Input: part model. Units: mm. Frame: model coordinates. Face numbers are marked on the shaded views. Round coordinates to 2 decimals unless told otherwise and drop trailing zeros. Loops run counter-clockwise (first coordinate to the right, second up) from the corner with the lowest first, then second, coordinate; pieces in that order, holes last. Notation, with made-up numbers: (57, -20) -> (75, -20) arc R28 cw to (75, 19) -> close; hole circle Ø1 at (39, 67.5). An arc over 180 degrees is marked (long way). Answer in a Markdown table with one row per item. Add a question column.
Q1. Section C-C, the plane x = 5.5. Output: boundary loops of the cut face in (y, z).
Q2. Pin query (flat end, axial travel): pin 1 (2.5 mm diameter, centred on x = 0.5, y = 1, fed in from +Z); pin 2 (6 mm diameter, centred on x = -10, y = -6.5, fed in from +Z); pin 3 (12 mm diameter, centred on x = -8.5, z = 38, fed in from -Y). Return the tip coordinate at first contact, or that it passes through.
Q3. Mould query, pull axis Z, two halves, no side actions, for the marked faces 1 and 2. Classes: pulls with the +Z half, pulls with the -Z half, needs draft (parallel to the pull), parting line crosses it, or undercut.
Q4. Section A-A, the plane y = 0. Output: boundary loops of the cut face in (x, z).
Q5. Ray query, L1, parallel to Z at x = -4, y = 12.5; L2, parallel to Z at x = 11.5, y = -2.5; L3, parallel to Z at x = -5.5, y = -5.5. Return the intervals inside material, ascending. Write a range as from..to.
Q6. Section D-D, the plane y = 4. Output: boundary loops of the cut face in (x, z), and give its area (3 significant figures).
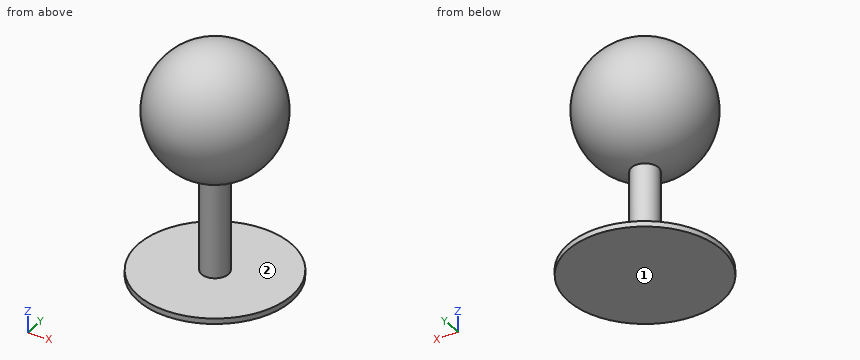
```python
from build123d import *

# Parameters (mm, degrees)
F0_R     = 15.380407463
F1_DEPTH = 1.1
F2_R     = 2.6884833656
F3_DEPTH = 32.2


with BuildPart() as f1:
    # F0 (on Top) → F1 (new body)
    with BuildSketch(Plane.XY):
        Circle(F0_R)
    extrude(amount=F1_DEPTH)

    # F2 (on face) → F3 (join)
    with BuildSketch(Plane.XY.offset(1.1)):
        Circle(F2_R)
    extrude(amount=F3_DEPTH)

    # F4 (on face) → F5 (revolve)
    with BuildSketch(Plane.XY.offset(33.3)):
        with BuildLine():
            Line((0, 2.6884833656), (0, 12.7))
            ThreePointArc((0, 12.7), (-12.7, 0), (0, -12.7))
            Line((0, -12.7), (0, -2.6884833656))
            ThreePointArc((0, -2.6884833656), (-2.6884833656, 0), (0, 2.6884833656))
        make_face()
    revolve(axis=Axis((0, 0, 33.3), (0, -1, 0)))


solid = f1.part
```
Answer block:
| question | item | result |
|---|---|---|
| 1 | outline | (-14.36, 0) -> (14.36, 0) -> (14.36, 1.1) -> (-14.36, 1.1) -> close; circle Ø22.89 at (0, 33.3) |
| 2 | pin 1 | z = 46 |
| 2 | pin 2 | z = 42.33 |
| 2 | pin 3 | y = -12.15 |
| 3 | face 1 | pulls with the -Z half |
| 3 | face 2 | undercut |
| 4 | outline | (-15.38, 0) -> (15.38, 0) -> (15.38, 1.1) -> (2.69, 1.1) -> (2.69, 20.89) arc R12.7 ccw (long way) to (-2.69, 20.89) -> (-2.69, 1.1) -> (-15.38, 1.1) -> close; hole (-2.69, 33.3) -> (2.69, 33.3) arc R2.69 ccw to start |
| 5 | L1 | 0..1.1 |
| 5 | L2 | 0..1.1, 28.53..38.07 |
| 5 | L3 | 0..1.1, 23.26..43.34 |
| 6 | outline | (-14.85, 0) -> (14.85, 0) -> (14.85, 1.1) -> (-14.85, 1.1) -> close; circle Ø24.11 at (0, 33.3) |
| 6 | area | 489 mm^2 |
